The figure shows three views and two pictorial views of one solid part (mm, origin at its lowest corner). Answer the questions. A direction names the side the tool comes from. Coordinates: 2 decimals unless noted, no trailing zeros. Loops run counter-clockwise (first coordinate to the right, second up) from the corner with the lowest first, then second, coordinate; pieces in that order, holes last. Notation, with made-up numbers: M 26.5,88 L 32.5,88 A33 cw 32.5,121 Z; hole C 86,12.5 d11. An arc over 180 degrees is marked long. One line per item, written item: value. Start each with the question number.
1. For the marked faces 1, 2 and 3, determine the directions among +Z, -Z, +X, -X, +Y, -Y from which every point of the face is accessible in a straight line to the end or side of a thin tool.
2. The part is cut by section B-B (z = 0.6). Write down the section's boundary in (x, y) (3 decimals), then the cut area to 3 significant figures.
3. The part is cut by section A-A (y = 1). Write down the section's boundary in (x, z) (3 decimals), then the cut area to 3 significant figures.
4. The part is cut by section C-C (x = 22). Write down the section's boundary in (y, z) (3 decimals).
5. Flat-ended cylindrical pins translate along their axes: pin 1 (1.6 mm diameter, centred on x = 38, z = 1.5, fed in from +Y) (3 decimals); pin 2 (0.9 mm diameter, centred on y = 8, z = 1.5, fed in from +X) (3 decimals); pin 3 (0.9 mm diameter, centred on x = 41, z = 1, fed in from -Y) (3 decimals); pin 4 (2 mm diameter, centred on x = 41, y = 2, fed in from +Z). Find the tip coordinate at first contact, or state that the pin passes through.
6. Consider probe 1 along X at (y, z) = (8.25, 1.5) (3 decimals); probe 2 along Y at (x, z) = (20.5, 0.8) (3 decimals). Determine where each line is inside the solid, lowest interval first.
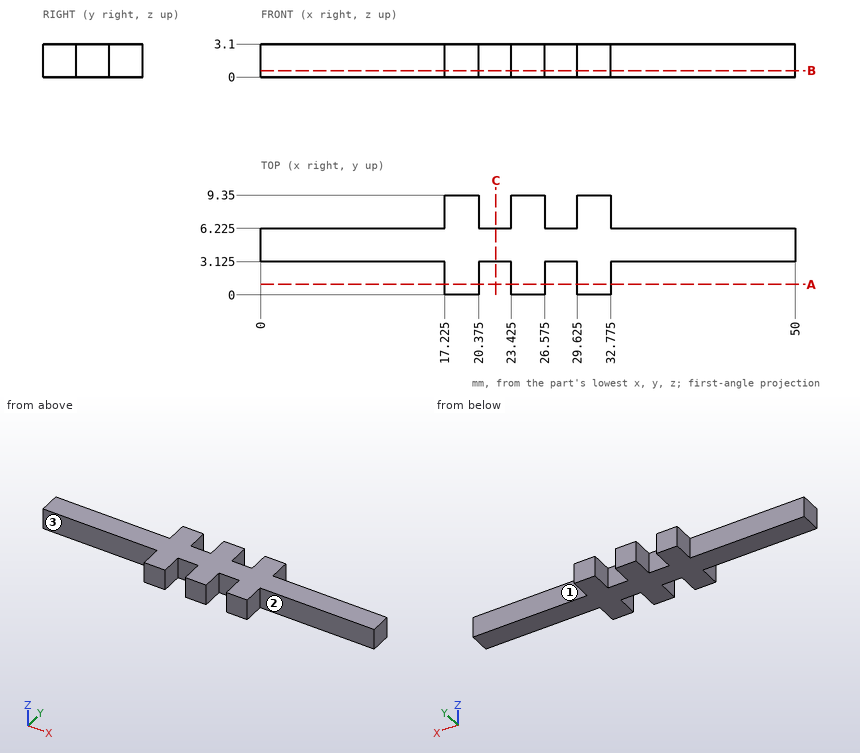
Answer block:
1. face 1: +Z, -Z, +X, +Y
1. face 2: +Z, -Z, +X, -Y
1. face 3: +Z, -Z, -X, -Y
2. outline: M 0,3.125 L 17.225,3.125 L 17.225,0 L 20.375,0 L 20.375,3.125 L 23.425,3.125 L 23.425,0 L 26.575,0 L 26.575,3.125 L 29.625,3.125 L 29.625,0 L 32.775,0 L 32.775,3.125 L 50,3.125 L 50,6.225 L 32.775,6.225 L 32.775,9.35 L 29.625,9.35 L 29.625,6.225 L 26.575,6.225 L 26.575,9.35 L 23.425,9.35 L 23.425,6.225 L 20.375,6.225 L 20.375,9.35 L 17.225,9.35 L 17.225,6.225 L 0,6.225 Z
2. area: 214 mm2
3. outline: M 17.225,0 L 20.375,0 L 20.375,3.1 L 17.225,3.1 Z; M 23.425,0 L 26.575,0 L 26.575,3.1 L 23.425,3.1 Z; M 29.625,0 L 32.775,0 L 32.775,3.1 L 29.625,3.1 Z
3. area: 29.3 mm2
4. outline: M 3.125,0 L 6.225,0 L 6.225,3.1 L 3.125,3.1 Z
5. pin 1: stops at y = 6.225
5. pin 2: stops at x = 32.775
5. pin 3: stops at y = 3.125
5. pin 4: passes through
6. probe 1: x = 17.225 to 20.375, 23.425 to 26.575, 29.625 to 32.775
6. probe 2: y = 3.125 to 6.225
